```python
from build123d import *

# Parameters (mm, degrees)
SKETCH1_W              = 25.4
SKETCH1_H              = 25.4
SKETCH1_W_2            = 19.05
SKETCH1_H_2            = 19.05
BOSS_EXTRUDE1_DEPTH    = 203.2
F_10_CLEARANCE_HOLE1_D = 5.1054


with BuildPart() as part:
    # Sketch1 → Boss-Extrude1 (new body)
    with BuildSketch(Plane.XY):
        with Locations((-12.7, 12.7)):
            Rectangle(SKETCH1_W, SKETCH1_H)
        with Locations((-12.7, 12.7)):
            Rectangle(SKETCH1_W_2, SKETCH1_H_2, mode=Mode.SUBTRACT)
    extrude(amount=BOSS_EXTRUDE1_DEPTH)

    # #10 Clearance Hole1 (through all)
    with Locations(Plane(origin=(0, 25.4, 0), x_dir=(1, 0, 0), z_dir=(0, 1, 0))):
        with Locations((-12.7, -165.1), (-12.7, -177.8), (-12.7, -190.5), (-12.7, -12.7), (-12.7, -25.4), (-12.7, -38.1)):
            Hole(F_10_CLEARANCE_HOLE1_D / 2)


solid = part.part
```
For this review, take the finished solid that the model builds, in its own axes (mm). A direction names the side the tool comes from. Round coordinates to 2 decimals unless told otherwise and drop trailing zeros. Write each loop counter-clockwise with the first axis right and the second up, starting at its lowest first coordinate (ties: lowest second). Pieces come first, ordered by that corner, then holes. Notation, with made-up numbers: (55, -1.5) - (83, -1.5) arc R29 cw to (83, 22.5) - close; hole circle Ø4 at (64, 56). An arc over 180 degrees is marked (long way). Use CSV: the item, a comma, the result in double quotes.
1) Add section B-B on x = -17.25. Write out the cut boundary in (y, z) (3 decimals).
Conclusion:
outline,"(0, 0) - (3.175, 0) - (3.175, 203.2) - (0, 203.2) - close; (22.225, 0) - (25.4, 0) - (25.4, 203.2) - (22.225, 203.2) - close"
2) Add section C-C on y = 8. Write out the cut boundary in (x, z) (3 decimals).
Conclusion:
outline,"(-25.4, 0) - (-22.225, 0) - (-22.225, 203.2) - (-25.4, 203.2) - close; (-3.175, 0) - (0, 0) - (0, 203.2) - (-3.175, 203.2) - close"
3) The part is to be moulded in two halves that separate along X. For faces 3 (the flat face through (-25.4, 13, 100)), 4 (the cylindrical face through (-12.147, 23.79, 192.992)), 5 (the flat face through (0, 13, 100)), 6 (the flat face through (-2, 13, 203.2)), say which applies: pulls with the +X half, pulls with the -X half, needs draft (parallel to the pull), parting line crosses it, or undercut.
Conclusion:
face 3,"pulls with the -X half"
face 4,"undercut"
face 5,"pulls with the +X half"
face 6,"needs draft"
4) For faces 1 (the flat face through (-22.225, 13, 100)), 2 (the cylindrical face through (-15.058, 23.79, 26.378)), list the 3-axis set-ups (+Z, -Z, +X, -X, +Y, -Y) from which the entire face can be reached by the end or side of a thin tool; tool diameter is ignored.
Conclusion:
face 1,"+Z, -Z"
face 2,"+Y, -Y"
5) Add section D-D on z = 12.7. Write out the cut boundary in (x, y) (3 decimals).
Conclusion:
outline,"(-25.4, 0) - (-15.253, 0) - (-15.253, 3.175) - (-22.225, 3.175) - (-22.225, 22.225) - (-15.253, 22.225) - (-15.253, 25.4) - (-25.4, 25.4) - close; (-10.147, 0) - (0, 0) - (0, 25.4) - (-10.147, 25.4) - (-10.147, 22.225) - (-3.175, 22.225) - (-3.175, 3.175) - (-10.147, 3.175) - close"
6) Wall thickness on line 1 along X through (y, z) = (14.75, 108.5) (3 decimals); line 2 along Y through (x, z) = (-5.5, 98) (3 decimals); line 3 along X through (y, z) = (1.4, 165.1): over which ranges is each line inside the solid? List them lowest first. Write a range as from..to.
Conclusion:
line 1,"x = -25.4..-22.225, -3.175..0"
line 2,"y = 0..3.175, 22.225..25.4"
line 3,"x = -25.4..-15.25, -10.15..0"
7) Add section A-A on z = 43. Write out the cut boundary in (x, y) (3 decimals).
Conclusion:
outline,"(-25.4, 0) - (0, 0) - (0, 25.4) - (-25.4, 25.4) - close; hole (-22.225, 3.175) - (-3.175, 3.175) - (-3.175, 22.225) - (-22.225, 22.225) - close"
